Read the model definition and answer for the solid it produces. Units are mm, in the model's axes. A direction names the side the tool comes from. Coordinates: 2 decimals unless noted, no trailing zeros. Write each loop counter-clockwise with the first axis right and the second up, starting at its lowest first coordinate (ties: lowest second). Pieces come first, ordered by that corner, then holes. Notation, with made-up numbers: (-11, 36.25) -> (45, 36.25) arc R18 cw to (45, 57.25) -> close; hole circle Ø10 at (5, 74). An arc over 180 degrees is marked (long way). Write item = value, one per line. Start each with the question number.
1) A tool of negligible diameter and unlimited length cuts with its end or side. For faces 5 (the face through (38, -16, 3.349)), 6 (the face through (37.64, -1.43, 4.85)), 7 (the face through (-32, -16, 20.094)), 8 (the face through (-82.379, -1.426, -6.279)), 9 (the face through (-31.312, -31.574, 21.597)), from which of +Z, -Z, +X, -X, +Y, -Y can it reach the whole face along a straight path? Write none if from no direction.
2) Section B-B (x = -47) is taken. Determine the outline of the cut face in (y, z).
3) Flat-ended cylindrical pins translate along their axes: pin 1 Ø3 at (x, y) = (38, -19.5) entering from -Z; pin 2 Ø3 at (x, y) = (46, -24.5) entering from -Z; pin 3 Ø12 at (x, y) = (10, -13.5) entering from -Z. Find the tip coordinate at first contact, or state that the pin passes through.
4) Find the intervals of material crossed by line 1 along X through (y, z) = (-11, 11.5); line 2 along X through (y, z) = (-21.5, 23); line 3 along X through (y, z) = (-31.5, 19) (3 decimals), in increasing order. Write a range as from..to.
5) Section A-A (y = -7.5) is taken. Determine the outline of the cut face in (x, z).
6) For a pull along X with two mould halves and no side action, classify faces 1 (the face through (22.839, -1.426, 12.866)), 2 (the face through (49.456, -16, 23)), 3 (the face through (-87.168, -16.661, -32.705)), 4 (the face through (52, -16, 8.349)) as released by +X, released by -X, zero draft, split by the parting line, or undercut.
from build123d import *

# Parameters (mm, degrees)
F1_DEPTH = 33
F2_F1_R  = 5
F2_F2_R  = 5


with BuildPart() as f1:
    # F0 (on Front) → F1 (new body)
    with BuildSketch(Plane.XZ):
        Polygon((44.3557138985, 43.3492468083), (-95.6442861015, 43.3492468083), (-95.6442861015, -33.8743397176), (-86.2685606181, -33.8743397176), (-75.6651710416, 20.0938743485), (9.3348289584, 20.0938743485), (34.3557138985, 3.3492468083), (44.3557138985, 3.3492468083), (44.3557138985, 37.0205976069), align=None)
        Polygon((54.3557138985, 43.3492468083), (44.3557138985, 43.3492468083), (44.3557138985, 37.0205976069), (49.4557138985, 37.0205976069), (49.4557138985, 8.3492468083), (54.3557138985, 8.3492468083), align=None)
    extrude(amount=F1_DEPTH)

    # F2: fillet of radius 5 on 19 edges, made by hand

    # F2_f1
    f2_f1_edges = [f1.edges().sort_by_distance(p)[0] for p in [
        (-75.6651710416, -16.5, 20.0938743485),
        (9.3348289584, -16.5, 20.0938743485),
    ]]
    fillet(f2_f1_edges, radius=F2_F1_R)

    # F2_f2
    f2_f2_edges = [f1.edges().sort_by_distance(p)[0] for p in [
        (-31.8679165952, 0, 20.0938743485),
        (-31.8679165952, -33, 20.0938743485),
        (-95.6442861015, -16.5, -33.8743397176),
        (-86.2685606181, -16.5, -33.8743397176),
        (-90.9564233598, 0, -33.8743397176),
        (-90.9564233598, -33, -33.8743397176),
        (-95.6442861015, -16.5, 43.3492468083),
        (-95.6442861015, 0, 4.7374535453),
        (-95.6442861015, -33, 4.7374535453),
        (-20.6442861015, 0, 43.3492468083),
        (-20.6442861015, -33, 43.3492468083),
        (34.3557138985, -16.5, 3.3492468083),
        (44.3557138985, -33, 20.1849222076),
        (44.3557138985, 0, 20.1849222076),
        (44.3557138985, -16.5, 3.3492468083),
        (39.3557138985, 0, 3.3492468083),
        (39.3557138985, -33, 3.3492468083),
        (-74.7284504953, -33, 18.9552032994),
        (9.2692742039, -33, 19.8780504751),
        (-74.7284504953, 0, 18.9552032994),
        (9.2692742039, 0, 19.8780504751),
    ]]
    fillet(f2_f2_edges, radius=F2_F2_R)


solid = f1.part
Answer key:
q1.face_5 = -Z, +X, +Y, -Y
q1.face_6 = -Z, +X, +Y
q1.face_7 = -Z, +Y, -Y
q1.face_8 = -Z, +Y
q1.face_9 = -Z, -Y
q2.outline = (-33, 25.09) arc R5 ccw to (-28, 20.09) -> (-5, 20.09) arc R5 ccw to (0, 25.09) -> (0, 38.35) arc R5 ccw to (-5, 43.35) -> (-28, 43.35) arc R5 ccw to (-33, 38.35) -> close
q3.pin_1 = 3.35
q3.pin_2 = 37.02
q3.pin_3 = 15.63
q4.line_1 = -95.64..-77.35, 22.18..44.36, 49.46..54.36
q4.line_2 = -95.64..44.36, 49.46..54.36
q4.line_3 = -94.215..-76.659, 13.539..42.926, 49.456..54.356
q5.outline = (-95.64, -28.87) arc R5 ccw to (-90.64, -33.87) -> (-90.38, -33.87) arc R5 ccw to (-85.48, -29.84) -> (-76.46, 16.06) arc R5 cw to (-71.55, 20.09) -> (7.82, 20.09) arc R5 cw to (10.6, 19.25) -> (33.09, 4.19) arc R5 ccw to (35.87, 3.35) -> (39.36, 3.35) arc R5 ccw to (44.36, 8.35) -> (44.36, 37.02) -> (49.46, 37.02) -> (49.46, 8.35) -> (54.36, 8.35) -> (54.36, 43.35) -> (-90.64, 43.35) arc R5 ccw to (-95.64, 38.35) -> close
q6.face_1 = undercut
q6.face_2 = undercut
q6.face_3 = released by +X
q6.face_4 = zero draft
